The listing builds one solid part. Answer for the finished solid, in the listing's coordinates (mm). A direction names the side the tool comes from. Coordinates: 2 decimals unless noted, no trailing zeros. Loops run counter-clockwise (first coordinate to the right, second up) from the corner with the lowest first, then second, coordinate; pieces in that order, holes last. Notation, with made-up numbers: (38, 6.5) - (95, 6.5) arc R28 cw to (95, 29.5) - close; hole circle Ø3 at (42, 54.5). An arc over 180 degrees is marked (long way). Use one line per item in the form item = value. Start each with the question number.
```python
from build123d import *

# Parameters (mm, degrees)
SKETCH1_W           = 19.5
SKETCH1_H           = 11.5
BOSS_EXTRUDE1_DEPTH = 8
FILLET1_R           = 2
SKETCH2_R           = 16.2
SKETCH2_R_2         = 14.7
CUT_EXTRUDE1_DEPTH  = 6
CUT_EXTRUDE2_REACH  = 13.5
SKETCH3_R           = 1.25
SKETCH4_W           = 6
SKETCH4_H           = 12.5
CUT_EXTRUDE3_DEPTH  = 9.0000001


with BuildPart() as part:
    # Sketch1 → Boss-Extrude1 (new body)
    with BuildSketch(Plane.XY):
        with Locations((0, 0.75)):
            Rectangle(SKETCH1_W, SKETCH1_H)
    extrude(amount=BOSS_EXTRUDE1_DEPTH)

    # Fillet1
    fillet1_edges = [part.edges().sort_by_distance(p)[0] for p in [
        (-9.75, 0.75, 8),
        (9.75, 0.75, 8),
    ]]
    fillet(fillet1_edges, radius=FILLET1_R)

    # Sketch2 → Cut-Extrude1 (cut)
    with BuildSketch(Plane.XY.offset(8)):
        with Locations((0, -16.2)):
            Circle(SKETCH2_R)
        with Locations((0, -16.2)):
            Circle(SKETCH2_R_2, mode=Mode.SUBTRACT)
    extrude(amount=-CUT_EXTRUDE1_DEPTH, mode=Mode.SUBTRACT)

    # Sketch3 → Cut-Extrude2 (cut, up to next)
    with BuildSketch(Plane(origin=(0, 6.5, 0), x_dir=(1, 0, 0), z_dir=(0, 1, 0)), mode=Mode.PRIVATE) as cut_extrude2_sk1:
        with Locations((5, -4)):
            Circle(SKETCH3_R)
    cut_extrude2_tool1 = extrude(cut_extrude2_sk1.sketch, amount=-CUT_EXTRUDE2_REACH, mode=Mode.PRIVATE) & part.part
    add(cut_extrude2_tool1.solids().sort_by_distance((5, 6.5, 4))[0], mode=Mode.SUBTRACT)
    # Sketch3 → Cut-Extrude2 (cut, up to next)
    with BuildSketch(Plane(origin=(0, 6.5, 0), x_dir=(1, 0, 0), z_dir=(0, 1, 0)), mode=Mode.PRIVATE) as cut_extrude2_sk2:
        with Locations((-5, -4)):
            Circle(SKETCH3_R)
    cut_extrude2_tool2 = extrude(cut_extrude2_sk2.sketch, amount=-CUT_EXTRUDE2_REACH, mode=Mode.PRIVATE) & part.part
    add(cut_extrude2_tool2.solids().sort_by_distance((-5, 6.5, 4))[0], mode=Mode.SUBTRACT)

    # Sketch4 → Cut-Extrude3 (cut, through all)
    with BuildSketch(Plane(origin=(0, 0, 0), x_dir=(-1, 0, 0), z_dir=(0, 0, -1))):
        with Locations((0, -5)):
            Rectangle(SKETCH4_W, SKETCH4_H)
    extrude(amount=-CUT_EXTRUDE3_DEPTH, mode=Mode.SUBTRACT)


solid = part.part
```
(1) For faces 4 (the face through (9.75, 1, 3)), 5 (the face through (-6.25, 2.68, 3.95)), 6 (the face through (0, 1.25, 4)), 7 (the face through (6.51, -3.02, 5.04)), determine the directions among +Z, -Z, +X, -X, +Y, -Y from which every point of the face is accessible in a straight line to the end or side of a thin tool.
(2) A cutting plane is placed at A-A (z = 2.5). Determine the outline of the cut face in (x, y).
(3) A cutting plane is placed at C-C (z = 4). Determine the outline of the cut face in (x, y), then the cut area to 3 significant figures.
(4) This flat-tipped pin is pushed along its axis until it touches: pin 1 Ø1.8 at (x, z) = (1.5, 5) entering from -Y. Where does it stop, or does it pass through?
(5) Determine the mould class of faces 1 (the face through (5, -4, 8)), 2 (the face through (8.36, -4.632, 7.905)), 3 (the face through (3, -2, 4)) for opening direction X: +X half, -X half, draft (parallel to the pull), parting line (faces both ways), or undercut.
(6) Find the intervals of material crossed by probe 1 along X at (y, z) = (2.5, 4); probe 2 along X at (y, z) = (-0.5, 1.25); probe 3 along X at (y, z) = (0.5, 4), in increasing order. Write a range as from..to.
(7) A cutting plane is placed at D-D (z = 0.5). Determine the outline of the cut face in (x, y).
(8) A cutting plane is placed at B-B (x = 4.25). Determine the outline of the cut face in (y, z).
Evaluation:
q1.face_4 = +Z, -Z, +X, +Y, -Y
q1.face_5 = +Y
q1.face_6 = +Z, -Z, -Y
q1.face_7 = +Z
q2.outline = (-9.75, -3.26) arc R16.2 cw to (-3, -0.28) - (-3, 1.25) - (3, 1.25) - (3, -0.28) arc R16.2 cw to (9.75, -3.26) - (9.75, 6.5) - (-9.75, 6.5) - close; (-9.52, -5) - (-3, -5) - (-3, -1.81) arc R14.7 ccw to start; (3, -5) - (9.52, -5) arc R14.7 ccw to (3, -1.81) - close
q3.outline = (-9.75, -3.26) arc R16.2 cw to (-6.25, -1.25) - (-6.25, 6.5) - (-9.75, 6.5) - close; (-9.52, -5) - (-3, -5) - (-3, -1.81) arc R14.7 ccw to start; (-3.75, -0.44) arc R16.2 cw to (-3, -0.28) - (-3, 1.25) - (3, 1.25) - (3, -0.28) arc R16.2 cw to (3.75, -0.44) - (3.75, 6.5) - (-3.75, 6.5) - close; (3, -5) - (9.52, -5) arc R14.7 ccw to (3, -1.81) - close; (6.25, -1.25) arc R16.2 cw to (9.75, -3.26) - (9.75, 6.5) - (6.25, 6.5) - close
q3.area = 128 mm^2
q4.pin_1 = 1.25
q5.face_1 = draft
q5.face_2 = +X half
q5.face_3 = undercut
q6.probe_1 = -9.75..-6.25, -3.75..3.75, 6.25..9.75
q6.probe_2 = -9.75..-3, 3..9.75
q6.probe_3 = -9.75..-6.25, -3.75..-3, 3..3.75, 6.25..9.75
q7.outline = (-9.75, -5) - (-3, -5) - (-3, 1.25) - (3, 1.25) - (3, -5) - (9.75, -5) - (9.75, 6.5) - (-9.75, 6.5) - close
q8.outline = (-5, 0) - (6.5, 0) - (6.5, 3) - (-0.57, 3) - (-0.57, 2) - (-2.13, 2) - (-2.13, 8) - (-5, 8) - close; (-0.57, 5) - (6.5, 5) - (6.5, 8) - (-0.57, 8) - close
